from build123d import *

# Parameters (mm, degrees)
F0_R     = 8.75
F1_DEPTH = 9


with BuildPart() as f1:
    # F0 (on Top) → F1 (new body)
    with BuildSketch(Plane.XY):
        with BuildLine():
            ThreePointArc((-55.6193343453, 33.109774836), (-52.0313924148, 41.7718329055), (-43.3693343453, 45.359774836))
            Line((-43.3693343453, 45.359774836), (-55.6193343453, 45.359774836))
            Line((-55.6193343453, 45.359774836), (-55.6193343453, 33.109774836))
        make_face()
        with BuildLine():
            Line((-55.6193343453, 21.200132486), (-43.7144180841, 20.8646363225))
            ThreePointArc((-43.7144180841, 20.8646363225), (-52.152550607, 24.570593839), (-55.6193343453, 33.109774836))
            Line((-55.6193343453, 33.109774836), (-55.6193343453, 21.200132486))
        make_face()
        with BuildLine():
            ThreePointArc((-43.7144180841, 20.8646363225), (-34.8301533483, 24.3265585742), (-31.1193343453, 33.109774836))
            ThreePointArc((-31.1193343453, 33.109774836), (-34.7072762757, 41.7718329055), (-43.3693343453, 45.359774836))
            ThreePointArc((-43.3693343453, 45.359774836), (-52.0313924148, 41.7718329055), (-55.6193343453, 33.109774836))
            ThreePointArc((-55.6193343453, 33.109774836), (-52.152550607, 24.570593839), (-43.7144180841, 20.8646363225))
        make_face()
        with Locations((-43.3693343453, 33.109774836)):
            Circle(F0_R, mode=Mode.SUBTRACT)
    extrude(amount=F1_DEPTH)


solid = f1.part
The model under review builds one solid part; all positions refer to its coordinate system, in mm. Give positions to 0.01 mm unless a question says otherwise; leave off trailing zeros. Loops run counter-clockwise (first coordinate to the right, second up) from the corner with the lowest first, then second, coordinate; pieces in that order, holes last. Notation, with made-up numbers: (34.25, 68.25) -> (60.25, 68.25) arc R16 ccw to (60.25, 91.25) -> close; hole circle Ø11 at (43.25, 89). An arc over 180 degrees is marked (long way). Put each result on its own line as item: value. Start each with the question number.
1. Mouldability with a two-part tool opening along X and no side actions: class faces 1 (the face through (-38.67, 40.49, 4.44)), 2 (the face through (-49, 45.36, 4)), 3 (the face through (-55.619, 33, 4)) as released by +X, released by -X, zero draft, split by the parting line, or undercut.
2. We need section A-A on x = -50.25. State the section outline as (y, z) points.
3. We need section B-B on y = 33.75. State the section outline as (x, z) points, then the cut area to 3 significant figures.
4. Clearance check with flat-ended pins moving along their axes: P1, Ø2, axis at x = -52, z = 1, coming from the -Y side; P2, Ø6, axis at x = -48.5, y = 35.5, coming from the +Z side; P3, Ø5, axis at x = -37.5, z = 3, coming from the -Y side. State where each tip first meets the part, or that it passes through.
5. Wall thickness on probe 1 along Y at (x, z) = (-43, 8); probe 2 along X at (y, z) = (33, 2); probe 3 along X at (y, z) = (26.75, 7.75): over which ranges is each line inside the solid? List them lowest first.
Determined:
1. face 1: undercut
1. face 2: zero draft
1. face 3: released by -X
2. outline: (21.05, 0) -> (27.7, 0) -> (27.7, 9) -> (21.05, 9) -> close; (38.52, 0) -> (45.36, 0) -> (45.36, 9) -> (38.52, 9) -> close
3. outline: (-55.62, 0) -> (-52.1, 0) -> (-52.1, 9) -> (-55.62, 9) -> close; (-34.64, 0) -> (-31.14, 0) -> (-31.14, 9) -> (-34.64, 9) -> close
3. area: 63.3 mm^2
4. P1: y = 21.07
4. P2: through
4. P3: y = 21.33
5. probe 1: 20.87 to 24.37, 41.85 to 45.35
5. probe 2: -55.62 to -52.12, -34.62 to -31.12
5. probe 3: -55.62 to -49.38, -37.36 to -32.9
